Verification items for the finished model (mm, model axes). A direction names the side the tool comes from. Round coordinates to 2 decimals unless told otherwise and drop trailing zeros. Loops run counter-clockwise (first coordinate to the right, second up) from the corner with the lowest first, then second, coordinate; pieces in that order, holes last. Notation, with made-up numbers: (15.25, 6.25) - (70.25, 6.25) arc R21 ccw to (70.25, 40.25) - close; hole circle Ø1 at (78, -8.5). An arc over 180 degrees is marked (long way). Use a Markdown table: item, result. Add a question column.
```python
from build123d import *

# Parameters (mm, degrees)
F1_ANGLE = 180


with BuildPart() as f1:
    # F0 (on Front) → F1 (revolve)
    with BuildSketch(Plane.XZ):
        Polygon((152.651871, 63.5), (-152.148129, 63.5), (-152.148129, 25.4), (-139.448129, 25.4), (-139.448129, 50.8), (-64.457401, 50.8), (-64.457401, 25.4), (-59.377401, 25.4), (-59.377401, 50.8), (40.299118, 50.8), (40.299118, 25.4), (45.379118, 25.4), (45.379118, 50.8), (140.436626, 50.8), (140.436626, 25.4), (153.136626, 25.4), align=None)
    revolve(axis=Axis((20.847701, 0, 0), (-1, 0, 0)), revolution_arc=F1_ANGLE)


solid = f1.part
```
Q1. Section check B-B on x = 103. Record the cut outline in (y, z), plus the area to 3 significant figures.
Q2. Go/stop test with flat-tipped pins: pin 1 Ø2 at (x, z) = (-121, 45.5) entering from +Y; pin 2 Ø12 at (x, z) = (-109, -45) entering from +Y; pin 3 Ø8 at (x, z) = (68, 9.5) entering from -Y. Record where each tip stops, or that it passes through.
Q3. Section check C-C on y = 28.5. State how many separate pieces and enclosed holes the cut face has, plus the area to 3 significant figures.
Q4. Release check for a two-part mould opening along Z. For faces 1 (the face through (-1.882, 63.485, 1.396)), 2 (the face through (-152.148, 32, -1)), 3 (the face through (-59.377, 26, 1)), 4 (the face through (-139.448, 26, 1)) record: +Z half, -Z half, draft (parallel to the pull), parting line (faces both ways), or undercut.
Q5. Section check A-A on z = 0. Record the cut outline in (x, y).
Q6. Thickness scan on line 1 along X through (y, z) = (29, -25.5); line 2 along X through (y, z) = (29, -5.5); line 3 along Z through (x, y) = (-56, 29.5). Record the ranges inside material, lowest first.
Q7. Set-up check for faces 5 (the face through (153.106, 27.777, 0.611)), 6 (the face through (-101.428, 50.788, 1.117)), 7 (the face through (146.876, 25.394, 0.559)): record each of +Z, -Z, +X, -X, +Y, -Y from which the full face is reachable in a straight line by a thin tool's end or side.
Determined:
| question | item | result |
|---|---|---|
| 1 | outline | (0, -63.5) arc R63.5 ccw to (0, 63.5) - (0, 50.8) arc R50.8 cw to (0, -50.8) - close |
| 1 | area | 2,280 mm² |
| 2 | pin 1 | stops at y = 45.3 |
| 2 | pin 2 | stops at y = 50.11 |
| 2 | pin 3 | stops at y = 48.97 |
| 3 | separate pieces | 1 |
| 3 | enclosed holes | 3 |
| 3 | area | 11,900 mm² |
| 4 | face 1 | parting line |
| 4 | face 2 | draft |
| 4 | face 3 | undercut |
| 4 | face 4 | undercut |
| 5 | outline | (-152.15, 25.4) - (-139.45, 25.4) - (-139.45, 50.8) - (-64.46, 50.8) - (-64.46, 25.4) - (-59.38, 25.4) - (-59.38, 50.8) - (40.3, 50.8) - (40.3, 25.4) - (45.38, 25.4) - (45.38, 50.8) - (140.44, 50.8) - (140.44, 25.4) - (153.14, 25.4) - (152.65, 63.5) - (-152.15, 63.5) - close |
| 6 | line 1 | x = -152.15 to -139.45, -64.46 to -59.38, 40.3 to 45.38, 140.44 to 152.97 |
| 6 | line 2 | x = -152.15 to -139.45, -64.46 to -59.38, 40.3 to 45.38, 140.44 to 153.08 |
| 6 | line 3 | z = -56.23 to -41.36, 41.36 to 56.23 |
| 7 | face 5 | +X, +Y |
| 7 | face 6 | -Y |
| 7 | face 7 | +X, -X, -Y |
